For this review, take the finished solid that the model builds, in its own axes (mm). Face numbers are marked on the shaded views. A direction names the side the tool comes from. Coordinates: 2 decimals unless noted, no trailing zeros. Write each loop counter-clockwise with the first axis right and the second up, starting at its lowest first coordinate (ties: lowest second). Pieces come first, ordered by that corner, then holes.
1) For the marked faces 1 and 2, list the 3-axis set-ups (+Z, -Z, +X, -X, +Y, -Y) from which the entire face can be reached by the end or side of a thin tool; tool diameter is ignored.
2) We need section D-D on z = -33.5. Write out the cut boundary in (x, y), then the cut area to 3 significant figures.
3) To check wall thickness, follow line 1 along X through (y, z) = (11.5, 0); line 2 along X through (y, z) = (2.25, -54); line 3 along X through (y, z) = (2.75, -67.5). State the ranges of each line that lie inside material, in increasing order.
4) Insertion check: P1, Ø8, axis at x = -28, y = 6.5, coming from the +Z side; P2, Ø1.2, axis at x = -0.5, z = 0.5, coming from the +Y side; P3, Ø6, axis at x = 7.5, z = -27, coming from the +Y side. Each pin has a flat end and moves straight along its axis. Give the tip position at first contact, or say it passes through.
5) We need section B-B on x = 63. Write out the cut boundary in (y, z), then the cut area to 3 significant figures.
6) We need section A-A on z = 68. Write out the cut boundary in (x, y).
7) We need section C-C on y = 9.5. Write out the cut boundary in (x, z), then the cut area to 3 significant figures.
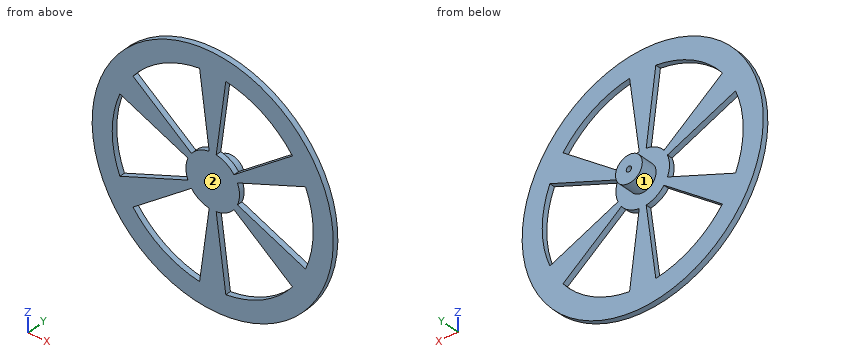
from build123d import *

# Parameters (mm, degrees)
SKETCH_1_R               = 90
EXTRUDE_1_DEPTH          = 4
CUT_EXTRUDE_1_DEPTH      = 128.342059038
PATTERN_CIRCULAR_1_COUNT = 6
SKETCH_6_R               = 10
EXTRUDE_2_DEPTH          = 12
SKETCH_7_R               = 2
CUT_EXTRUDE_2_DEPTH      = 12


with BuildPart() as part:
    # Sketch 1 → Extrude 1 (new body)
    with BuildSketch(Plane(origin=(0, 0, 0), x_dir=(1, 0, 0), z_dir=(0, 1, 0))):
        with Locations(Location((0, 0, 0), (0, 0, 270))):
            Circle(SKETCH_1_R)
    extrude(amount=EXTRUDE_1_DEPTH)

    # Sketch 2 → Cut-Extrude 1 (cut, through all)
    with BuildSketch(Plane(origin=(0, 4, 0), x_dir=(1, 0, 0), z_dir=(0, 1, 0))):
        with BuildLine():
            ThreePointArc((-15.867066806, 12.17522858), (-10, 17.320508076), (-2.610523844, 19.828897227))
            Line((-2.610523844, 19.828897227), (-9.789464417, 74.358364603))
            ThreePointArc((-9.789464417, 74.358364603), (-37.5, 64.951905284), (-59.501500522, 45.657107176))
            Line((-59.501500522, 45.657107176), (-15.867066806, 12.17522858))
        make_face()
    cut_extrude_1 = extrude(amount=-CUT_EXTRUDE_1_DEPTH, mode=Mode.SUBTRACT)

    # Pattern Circular 1: Cut-Extrude 1 ×6 about axis
    pattern_circular_1_axis = Axis((0, 0, 0), (0, 1, 0))
    for i in range(1, PATTERN_CIRCULAR_1_COUNT):
        add(cut_extrude_1.rotate(pattern_circular_1_axis, i * 360 / PATTERN_CIRCULAR_1_COUNT), mode=Mode.SUBTRACT)

    # Sketch 6 → Extrude 2 (add)
    with BuildSketch(Plane(origin=(0, 4, 0), x_dir=(1, 0, 0), z_dir=(0, 1, 0))):
        with Locations(Location((0, 0, 0), (0, 0, 270))):
            Circle(SKETCH_6_R)
    extrude(amount=EXTRUDE_2_DEPTH)

    # Sketch 7 → Cut-Extrude 2 (cut)
    with BuildSketch(Plane(origin=(0, 16, 0), x_dir=(1, 0, 0), z_dir=(0, 1, 0))):
        with Locations(Location((0, 0, 0), (0, 0, 270))):
            Circle(SKETCH_7_R)
    extrude(amount=-CUT_EXTRUDE_2_DEPTH, mode=Mode.SUBTRACT)


solid = part.part
Result:
1. face 1: +Y
1. face 2: +Z, -Z, +X, -X, -Y
2. outline: (-83.53, 0) - (-43.66, 0) - (-43.66, 4) - (-83.53, 4) - close; (-4.41, 0) - (4.41, 0) - (4.41, 4) - (-4.41, 4) - close; (43.66, 0) - (83.53, 0) - (83.53, 4) - (43.66, 4) - close
2. area: 354 mm2
3. line 1: x = -10 to -2, 2 to 10
3. line 2: x = -72 to -52.05, -7.11 to 7.11, 52.05 to 72
3. line 3: x = -59.53 to -32.69, -8.89 to 8.89, 32.69 to 59.53
4. P1: stops at z = 86.49
4. P2: stops at y = 4
4. P3: passes through
5. outline: (0, -64.27) - (4, -64.27) - (4, -26.1) - (0, -26.1) - close; (0, 26.1) - (4, 26.1) - (4, 64.27) - (0, 64.27) - close
5. area: 305 mm2
6. outline: (-58.96, 0) - (-31.64, 0) - (-31.64, 4) - (-58.96, 4) - close; (-8.95, 0) - (8.95, 0) - (8.95, 4) - (-8.95, 4) - close; (31.64, 0) - (58.96, 0) - (58.96, 4) - (31.64, 4) - close
7. outline: circle Ø20 at (0, 0); hole circle Ø4 at (0, 0)
7. area: 302 mm2
